Build history of the part. All positions in model axes, mm. Give positions to 0.01 mm unless a question says otherwise; leave off trailing zeros. Write each loop counter-clockwise with the first axis right and the second up, starting at its lowest first coordinate (ties: lowest second). Pieces come first, ordered by that corner, then holes. Notation, with made-up numbers: (52.5, 45) -> (104.5, 45) arc R26 ccw to (104.5, 80) -> close; hole circle Ø4 at (81, 56). An arc over 180 degrees is marked (long way). Write item = value, one per line. Start each with the question number.
Q1. Drop flat-ended pins along their axis: P1, Ø10, axis at x = -10.5, y = 37.5, coming from the +Z side; P2, Ø4, axis at x = -45.51, y = 38.51, coming from the +Z side (3 decimals). Give the stop position or say it passes through.
Q2. Saw through at C-C, the plane y = 33.5. List the corners of the cut face in (x, z), then the cut area to 3 significant figures.
Q3. Saw through at B-B, the plane x = -14.5. List the corners of the cut face in (y, z), then the cut area to 3 significant figures.
Q4. Wall check: line 1 (X direction, y = 37, z = 1.3); line 2 (Y direction, x = -46, z = 1.2); line 3 (Y direction, x = -8, z = 1.7). Give the ranges that are in metal, low to high.
from build123d import *

# Parameters (mm, degrees)
F0_R      = 2.38125
F1_DEPTH  = 2.38125
F2_R      = 7.9375
F4_DEPTH  = 19.051
F6_DEPTH  = 9.5648146833
F8_DEPTH  = 19.051
F10_DEPTH = 60.326


with BuildPart() as f1:
    # F0 (on Top) → F1 (new body)
    with BuildSketch(Plane.XY):
        with BuildLine():
            Line((6.8802531183, 46.4430405467), (-53.4447468817, 46.4430405467))
            Line((-53.4447468817, 46.4430405467), (-53.4447468817, 27.3930405467))
            Line((-53.4447468817, 27.3930405467), (-43.9197468817, 27.3930405467))
            Line((-43.9197468817, 27.3930405467), (-41.3273820942, 35.0202070092))
            ThreePointArc((-41.3273820942, 35.0202070092), (-40.0228140496, 36.8628863815), (-37.9243791103, 37.6959145069))
            Line((-37.9243791103, 37.6959145069), (6.8802531183, 40.0930405467))
            Line((6.8802531183, 40.0930405467), (6.8802531183, 46.4430405467))
        make_face()
        with Locations((-45.5072468817, 38.5055405467)):
            Circle(F0_R, mode=Mode.SUBTRACT)
    extrude(amount=F1_DEPTH)

    # F2
    f2_edges = [f1.edges().sort_by_distance(p)[0] for p in [
        (-53.444747, 46.443041, 1.190625),
    ]]
    fillet(f2_edges, radius=F2_R)

    # F3 (on face) → F4 (cut, through all)
    with BuildSketch(Plane(origin=(0, 46.4430405467, 0), x_dir=(-1, 0, 0), z_dir=(0, 1, 0))):
        Polygon((-7.2697603085, 1.5504802494), (-6.8802531183, 1.5907407505), (8.2211783156, 2.38125), (8.2030607001, 2.727358446), (-7.2193359956, 3.1990723219), align=None)
    extrude(amount=-F4_DEPTH, mode=Mode.SUBTRACT)

    # F5 (on face) → F6 (cut, through all)
    with BuildSketch(Plane(origin=(-2.1192870449, 39.6115494375, 0), x_dir=(0.9985718469, 0.053425337, 0), z_dir=(0.053425337, -0.9985718469, 0))):
        Polygon((9.0124112666, 0.7953703753), (-6.0780490749, 0), (9.0124112666, 0), align=None)
    extrude(amount=-F6_DEPTH, mode=Mode.SUBTRACT)

    # F7 (on face) → F8 (cut, through all)
    with BuildSketch(Plane(origin=(0, 46.4430405467, 0), x_dir=(-1, 0, 0), z_dir=(0, 1, 0))):
        Polygon((-6.5405170331, 0.7953703753), (-6.8802531183, 0.7953703753), (-6.9836541079, 0.7953703753), (-6.9836541079, -0.0977396412), (-6.5405170331, -0.0977396412), align=None)
    extrude(amount=-F8_DEPTH, mode=Mode.SUBTRACT)

    # F9 (on face) → F10 (cut, through all)
    with BuildSketch(Plane(origin=(-53.4447468817, 0, 0), x_dir=(0, -1, 0), z_dir=(-1, 0, 0))):
        Polygon((-35.3305405467, 2.38125), (-27.3930405467, 1.984375), (-26.6849351877, 1.984375), (-26.7145372927, 2.7254258748), align=None)
        Polygon((-26.9428193569, 0.396875), (-27.3930405467, 0.396875), (-35.3432405467, 0), (-35.0132025778, -0.3093605337), (-26.8219634891, -0.3093605337), align=None)
    extrude(amount=-F10_DEPTH, mode=Mode.SUBTRACT)


solid = f1.part
Report:
q1.P1 = 2.38
q1.P2 = through
q2.outline = (-53.44, 0.09) -> (-41.84, 0.09) -> (-41.84, 2.29) -> (-53.44, 2.29) -> close
q2.area = 25.5 mm2
q3.outline = (38.95, 0) -> (46.44, 0) -> (46.44, 2.38) -> (38.95, 2.38) -> close
q3.area = 17.8 mm2
q4.line_1 = -53.44 to -47.35, -43.66 to -39.84
q4.line_2 = 27.39 to 36.18, 40.84 to 46.43
q4.line_3 = 39.3 to 46.44
